```python
from build123d import *

# Parameters (mm, degrees)
F1_W     = 355.6
F1_H     = 435.326967
F2_DEPTH = 19.05
F3_DEPTH = 19.051


with BuildPart() as f2:
    # F1 (on Top) → F2 (new body)
    with BuildSketch(Plane.XY):
        with Locations((0, -217.663483)):
            Rectangle(F1_W, F1_H)
    extrude(amount=-F2_DEPTH)

    # F0 (on Top) → F3 (cut, through all)
    with BuildSketch(Plane.XY):
        with BuildLine():
            ThreePointArc((-97.080427, -116.062633), (-76.2, -127), (-55.319573, -116.062633))
            ThreePointArc((-55.319573, -116.062633), (-28.328574, -60.798883), (-19.05, 0))
            ThreePointArc((-19.05, 0), (-76.2, 57.15), (-133.35, 0))
            ThreePointArc((-133.35, 0), (-124.071426, -60.798883), (-97.080427, -116.062633))
        make_face()
        with BuildLine():
            ThreePointArc((19.05, 0), (28.328574, -60.798883), (55.319573, -116.062633))
            ThreePointArc((55.319573, -116.062633), (76.2, -127), (97.080427, -116.062633))
            ThreePointArc((97.080427, -116.062633), (124.071426, -60.798883), (133.35, 0))
            ThreePointArc((133.35, 0), (76.2, 57.15), (19.05, 0))
        make_face()
    extrude(amount=-F3_DEPTH, mode=Mode.SUBTRACT)


solid = f2.part
```
Geometry check sheet. Reference: the model listing, model coordinates, mm. A direction names the side the tool comes from. Give positions to 0.01 mm unless a question says otherwise; leave off trailing zeros. Loops run counter-clockwise (first coordinate to the right, second up) from the corner with the lowest first, then second, coordinate; pieces in that order, holes last. Notation, with made-up numbers: M -26.5,57.5 L 30.5,57.5 A8 ccw 30.5,68.5 Z; hole C 12.5,18 d4. An arc over 180 degrees is marked long. Write item = value, one per line.
(1) Sectioned sample at B-B, the plane z = -14. Record the cut outline in (x, y) (3 decimals).
Answer below:
outline = M -177.8,-435.327 L 177.8,-435.327 L 177.8,0 L 133.35,0 A203.835 cw 97.08,-116.063 A25.4 cw 55.32,-116.063 A203.835 cw 19.05,0 L -19.05,0 A203.835 cw -55.32,-116.063 A25.4 cw -97.08,-116.063 A203.835 cw -133.35,0 L -177.8,0 Z
(2) Sectioned sample at D-D, the plane y = -54. Record the cut outline in (x, z), plus the area to 3 significant figures.
Answer below:
outline = M -177.8,-19.05 L -126.07,-19.05 L -126.07,0 L -177.8,0 Z; M -26.33,-19.05 L 26.33,-19.05 L 26.33,0 L -26.33,0 Z; M 126.07,-19.05 L 177.8,-19.05 L 177.8,0 L 126.07,0 Z
area = 2,970 mm2
(3) Gauge pin test, flat end, axial feed: pin 1 Ø3 at (x, y) = (-8, -51.5) entering from +Z. Record the tip position at first contact, or that the pin passes through.
Answer below:
pin_1 = 0
(4) Release check for a two-part mould opening along X. For faces 3 (the face through (177.8, -221, -9)), 4 (the face through (76, -127, -9)), 5 (the face through (-177.8, -221, -9)), 6 (the face through (-124.33, -59.97, -9.39)) record: released by +X, released by -X, zero draft, split by the parting line, or undercut.
Answer below:
face_3 = released by +X
face_4 = undercut
face_5 = released by -X
face_6 = undercut
(5) Sectioned sample at A-A, the plane y = -105.5. Record the cut outline in (x, z), plus the area to 3 significant figures.
Answer below:
outline = M -177.8,-19.05 L -103.92,-19.05 L -103.92,0 L -177.8,0 Z; M -48.48,-19.05 L 48.48,-19.05 L 48.48,0 L -48.48,0 Z; M 103.92,-19.05 L 177.8,-19.05 L 177.8,0 L 103.92,0 Z
area = 4,660 mm2
(6) Tool access check on faces 1 (the face through (-156, 0, -9)), 2 (the face through (-28.588, -61.623, -9.392)). Record the directions out of +Z, -Z, +X, -X, +Y, -Y that give a thin tool (end or side, any length) a straight path to the whole face; none if there is none.
Answer below:
face_1 = +Z, -Z, +X, -X, +Y
face_2 = +Z, -Z, +Y
(7) Material ranges on line 1 (X direction, y = -100, z = -3.5); line 2 (X direction, y = -43, z = -12.25); line 3 (Y direction, x = 65.5, z = -2.75), recorded low to high. Write a range as [from, to].
Answer below:
line_1 = [-177.8, -107.13], [-45.27, 45.27], [107.13, 177.8]
line_2 = [-177.8, -128.76], [-23.64, 23.64], [128.76, 177.8]
line_3 = [-435.33, -124.64]
(8) Sectioned sample at C-C, the plane x = 36. Record the cut outline in (y, z), plus the area to 3 significant figures.
Answer below:
outline = M -435.33,-19.05 L -81.38,-19.05 L -81.38,0 L -435.33,0 Z
area = 6,740 mm2
